Verification items for this drawing (mm, ordinates from the low corner). A direction names the side the tool comes from. Coordinates: 2 decimals unless noted, no trailing zeros. Write each loop counter-clockwise with the first axis right and the second up, starting at its lowest first coordinate (ties: lowest second). Pieces come first, ordered by that corner, then holes.
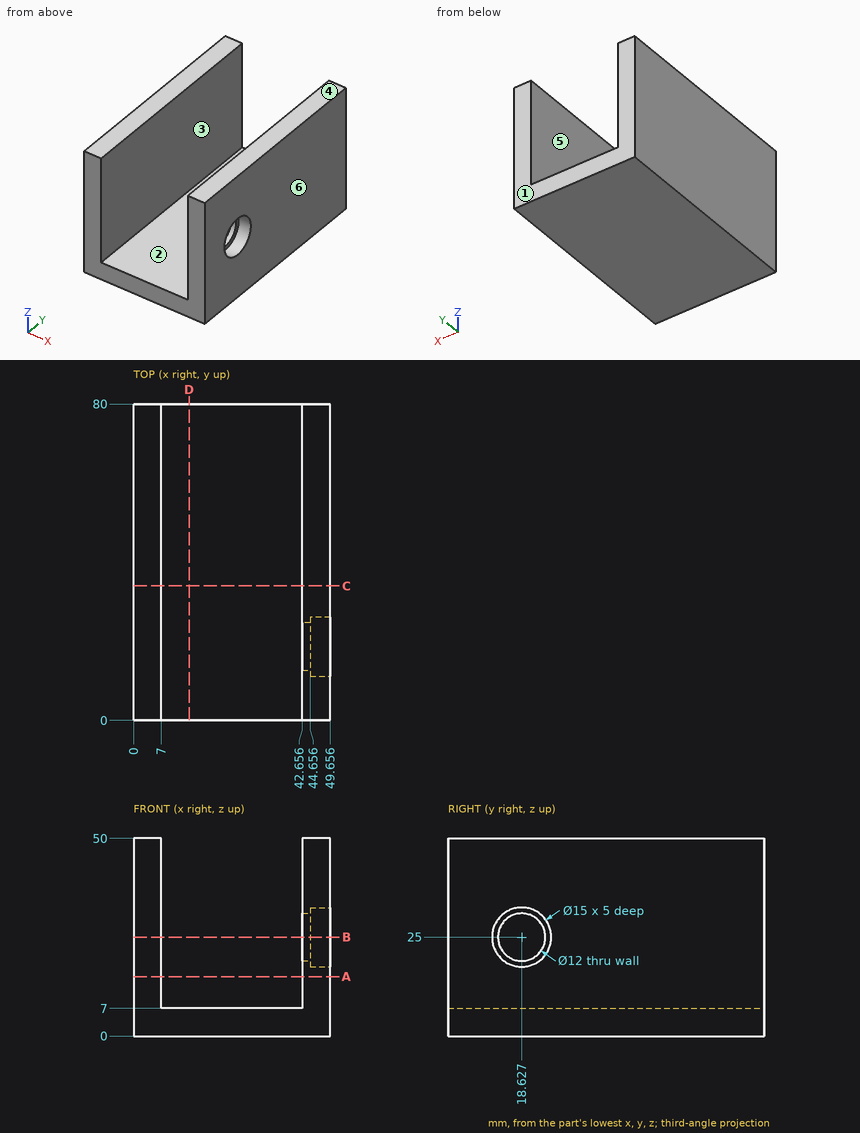
1. Gauge pin test, flat ends, axial feed: pin 1 Ø5 at (y, z) = (22, 27.5) entering from +X; pin 2 Ø10 at (x, y) = (30, 46) entering from +Z; pin 3 Ø9 at (y, z) = (18.63, 25) entering from +X. Record the tip position at first contact, or that the pin passes through.
Computed values:
pin 1: stops at x = 44.66
pin 2: stops at z = 7
pin 3: stops at x = 7
2. Thickness scan on line 1 along X through (y, z) = (38, 10); line 2 along Z through (x, y) = (32.5, 62). Record the ranges inside material, lowest first.
Computed values:
line 1: x = 0 to 7, 42.66 to 49.66
line 2: z = 0 to 7
3. Sectioned sample at A-A, the plane z = 15. Record the boundary of the cut face in (x, y), and give its area (3 significant figures).
Computed values:
outline: (0, 0) - (7, 0) - (7, 80) - (0, 80) - close; (42.66, 0) - (49.66, 0) - (49.66, 80) - (42.66, 80) - close
area: 1,120 mm2
4. Access from +Z, -Z, +X, -X, +Y, -Y to the whole of each face (thin tool, end or side, straight path). Record for the marked faces 1 and 2.
Computed values:
face 1: +Z, -Z, +X, -X, +Y
face 2: +Z, +Y, -Y
5. Sectioned sample at D-D, the plane x = 14. Record the boundary of the cut face in (y, z), and give its area (3 significant figures).
Computed values:
outline: (0, 0) - (80, 0) - (80, 7) - (0, 7) - close
area: 560 mm2
6. Sectioned sample at C-C, the plane y = 34. Record the boundary of the cut face in (x, z).
Computed values:
outline: (0, 0) - (49.66, 0) - (49.66, 50) - (42.66, 50) - (42.66, 7) - (7, 7) - (7, 50) - (0, 50) - close
7. Draft check along X on the marked faces 3, 4, 5 and 6. Enter one of: released by +X, released by -X, zero draft, split by the parting line, or undercut.
Computed values:
face 3: undercut
face 4: zero draft
face 5: undercut
face 6: released by +X
8. Sectioned sample at B-B, the plane z = 25. Record the boundary of the cut face in (x, y), and give its area (3 significant figures).
Computed values:
outline: (0, 0) - (7, 0) - (7, 80) - (0, 80) - close; (42.66, 0) - (49.66, 0) - (49.66, 11.13) - (44.66, 11.13) - (44.66, 12.63) - (42.66, 12.63) - close; (42.66, 24.63) - (44.66, 24.63) - (44.66, 26.13) - (49.66, 26.13) - (49.66, 80) - (42.66, 80) - close
area: 1,020 mm2
